```python
from build123d import *

# Parameters (mm, degrees)
CUT_EXTRUDE_1_DEPTH      = 10
HOLE_WIZARD_M2_5_1_D     = 2.05
HOLE_WIZARD_M2_5_1_DEPTH = 6.35
HOLE_WIZARD_M2_5_1_TIP   = 0.615882135
HOLE_WIZARD_M2_1_D       = 1.6
HOLE_WIZARD_M2_1_DEPTH   = 5.2
HOLE_WIZARD_M2_1_TIP     = 0.480688495


with BuildPart() as part:
    # 草图1 → 旋转1 (revolve)
    with BuildSketch(Plane.XY):
        Polygon((0, 0), (4, 0), (4, 3), (1.5, 3), (1.5, 6), (11, 6), (11, 80.5), (6, 80.5), (6, 82.5), (2, 82.5), (2, 95), (0, 95), align=None)
    revolve(axis=Axis((0, 0, 0), (0, 1, 0)))

    # 草图2 → 切除-拉伸1 (cut)
    with BuildSketch(Plane(origin=(0, 95, 0), x_dir=(1, 0, 0), z_dir=(0, 1, 0))):
        with BuildLine():
            Line((-1.15, -1.636306817), (-1.15, 1.636306817))
            ThreePointArc((-1.15, 1.636306817), (-2, 0), (-1.15, -1.636306817))
        make_face()
        with BuildLine():
            ThreePointArc((2, 0), (1.774823935, 0.921954446), (1.15, 1.636306817))
            Line((1.15, 1.636306817), (1.15, -1.636306817))
            ThreePointArc((1.15, -1.636306817), (1.774823935, -0.921954446), (2, 0))
        make_face()
    extrude(amount=-CUT_EXTRUDE_1_DEPTH, mode=Mode.SUBTRACT)

    # M2.5 螺纹孔1
    with Locations(Plane(origin=(0, 80.5, 0), x_dir=(1, 0, 0), z_dir=(0, 1, 0))):
        with Locations((0, 8.660254038), (-7.5, -4.330127019), (7.5, -4.330127019)):
            Hole(HOLE_WIZARD_M2_5_1_D / 2, depth=HOLE_WIZARD_M2_5_1_DEPTH)
            with Locations((0, 0, -(HOLE_WIZARD_M2_5_1_DEPTH + HOLE_WIZARD_M2_5_1_TIP / 2))):  # 118° drill point
                Cone(0, HOLE_WIZARD_M2_5_1_D / 2, HOLE_WIZARD_M2_5_1_TIP, mode=Mode.SUBTRACT)

    # M2 螺纹孔1
    with Locations(Plane(origin=(0, 6, 0), x_dir=(-1, 0, 0), z_dir=(0, -1, 0))):
        with Locations((-6.5, 0), (6.5, 0)):
            Hole(HOLE_WIZARD_M2_1_D / 2, depth=HOLE_WIZARD_M2_1_DEPTH)
            with Locations((0, 0, -(HOLE_WIZARD_M2_1_DEPTH + HOLE_WIZARD_M2_1_TIP / 2))):  # 118° drill point
                Cone(0, HOLE_WIZARD_M2_1_D / 2, HOLE_WIZARD_M2_1_TIP, mode=Mode.SUBTRACT)


solid = part.part
```
Can you work these out from the model? Positions are in its coordinate system, mm. A direction names the side the tool comes from. Round coordinates to 2 decimals unless told otherwise and drop trailing zeros. Loops run counter-clockwise (first coordinate to the right, second up) from the corner with the lowest first, then second, coordinate; pieces in that order, holes last.
Item 1: If we mould it in two halves opening along Z, with no side actions, what happens to faces 1 (the flat face through (-1.15, 90, 0)), 2 (the conical face through (-6.39, 11.6, 0.08)), 3 (the cylindrical face through (0.923, 87.449, 1.774))? For each: +Z half, -Z half, draft (parallel to the pull), parting line (faces both ways), or undercut.
Item 2: Which directions (+Z, -Z, +X, -X, +Y, -Y) give clear straight access to the entire face, cutting with the end or side of a thin tool? Please do faces 4 (the cylindrical face through (5.7, 8.6, 0)), 5 (the cylindrical face through (-6.476, 77.281, 4.285)), 6 (the flat face through (2, 3, 0)), 7 (the flat face through (1.15, 90, 0)), 8 (the cylindrical face through (-2.38, 43.77, 10.74)).
Item 3: Suppose I cut it at C-C, the plane z = 8.75. Write out the boundary of the cut face in (x, y), then the cut area to 3 significant figures.
Item 4: Please list where these lines run through material, in increasing order: L1, parallel to Y at x = -1.5, z = 1.5; L2, parallel to Z at x = 0, y = 78.25; L3, parallel to Y at x = 3, z = -7.5.
Item 5: Suppose I cut it at B-B, the plane y = 70. Write out the boundary of the cut face in (x, z).
Item 6: Suppose I cut it at A-A, the plane y = 8. Write out the boundary of the cut face in (x, z).
Item 7: Will these pins go through, and if not, where does the flat tip stop? pin 1 Ø2.5 at (y, z) = (90, 0.5) entering from -X; pin 2 Ø1.5 at (x, z) = (7.5, 2.5) entering from -Y; pin 3 Ø10 at (x, y) = (-5.5, 53) entering from -Z.
Reported:
1. face 1: draft
1. face 2: undercut
1. face 3: parting line
2. face 4: -Y
2. face 5: +Y
2. face 6: none
2. face 7: +Z, -Z, +X, +Y
2. face 8: +Y, -Y
3. outline: (-6.67, 6) - (6.67, 6) - (6.67, 80.5) - (-6.67, 80.5) - close
3. area: 993 mm2
4. L1: y = 0 to 3, 6 to 82.5
4. L2: z = -11 to -9.69, -7.64 to 11
4. L3: y = 6 to 80.5
5. outline: circle Ø22 at (0, 0)
6. outline: circle Ø22 at (0, 0); hole circle Ø1.6 at (-6.5, 0); hole circle Ø1.6 at (6.5, 0)
7. pin 1: stops at x = -1.15
7. pin 2: stops at y = 6
7. pin 3: stops at z = -10.99
